```python
from build123d import *

# Parameters (mm, degrees)
SKETCH1_W           = 90
SKETCH1_H           = 70
BOSS_EXTRUDE1_DEPTH = 4
SKETCH2_R           = 1.75
CUT_EXTRUDE1_DEPTH  = 5
CHAMFER1_SIZE       = 2
CHAMFER2_SIZE       = 2
CHAMFER3_SIZE       = 2
CHAMFER4_SIZE       = 2
SKETCH5_W           = 70
SKETCH5_H           = 4
BOSS_EXTRUDE3_DEPTH = 10
SKETCH4_W           = 70
SKETCH4_H           = 4
BOSS_EXTRUDE4_DEPTH = 10
SKETCH6_R           = 1.75
CUT_EXTRUDE2_DEPTH  = 10
CHAMFER5_SIZE       = 2
SKETCH7_W           = 40
SKETCH7_H           = 40
CUT_EXTRUDE3_DEPTH  = 2
SKETCH8_W           = 25
SKETCH8_H           = 15
CUT_EXTRUDE4_DEPTH  = 2
SKETCH9_R           = 1.5
CUT_EXTRUDE5_DEPTH  = 4
SKETCH10_R          = 1.75
CUT_EXTRUDE6_DEPTH  = 10


with BuildPart() as part:
    # Sketch1 → Boss-Extrude1 (new body)
    with BuildSketch(Plane.XY):
        with Locations((44.768273235, 35.193370166)):
            Rectangle(SKETCH1_W, SKETCH1_H)
    extrude(amount=BOSS_EXTRUDE1_DEPTH)

    # Sketch2 → Cut-Extrude1 (cut)
    with BuildSketch(Plane.XY.offset(4)):
        with Locations((3.703568783, 2.693370166)):
            Circle(SKETCH2_R)
        with Locations((86.703568783, 2.694436567)):
            Circle(SKETCH2_R)
        with Locations((86.703273235, 67.693370166)):
            Circle(SKETCH2_R)
        with Locations((3.703273235, 67.693370166)):
            Circle(SKETCH2_R)
        with Locations((23.297725672, 13.693370166)):
            Circle(SKETCH2_R)
        with Locations((66.284051901, 13.693370166)):
            Circle(SKETCH2_R)
        with Locations((66.268273235, 56.693370166)):
            Circle(SKETCH2_R)
        with Locations((23.268273235, 56.693370166)):
            Circle(SKETCH2_R)
    extrude(amount=-CUT_EXTRUDE1_DEPTH, mode=Mode.SUBTRACT)

    # Chamfer1
    chamfer1_edges = [part.edges().sort_by_distance(p)[0] for p in [
        (89.768273235, 0.193370166, 2),
    ]]
    chamfer(chamfer1_edges, length=CHAMFER1_SIZE)

    # Chamfer2
    chamfer2_edges = [part.edges().sort_by_distance(p)[0] for p in [
        (-0.231726765, 0.193370166, 2),
    ]]
    chamfer(chamfer2_edges, length=CHAMFER2_SIZE)

    # Chamfer3
    chamfer3_edges = [part.edges().sort_by_distance(p)[0] for p in [
        (-0.231726765, 70.193370166, 2),
    ]]
    chamfer(chamfer3_edges, length=CHAMFER3_SIZE)

    # Chamfer4
    chamfer4_edges = [part.edges().sort_by_distance(p)[0] for p in [
        (89.768273235, 70.193370166, 2),
    ]]
    chamfer(chamfer4_edges, length=CHAMFER4_SIZE)

    # Sketch5 → Boss-Extrude3 (add)
    with BuildSketch(Plane(origin=(0, 70.193370166, 0), x_dir=(1, 0, 0), z_dir=(0, 1, 0))):
        with Locations((44.768273235, -2)):
            Rectangle(SKETCH5_W, SKETCH5_H)
    extrude(amount=BOSS_EXTRUDE3_DEPTH)

    # Sketch4 → Boss-Extrude4 (add)
    with BuildSketch(Plane(origin=(0, 0.193370166, 0), x_dir=(-1, 0, 0), z_dir=(0, -1, 0))):
        with Locations((-44.768273235, -2)):
            Rectangle(SKETCH4_W, SKETCH4_H)
    extrude(amount=BOSS_EXTRUDE4_DEPTH)

    # Sketch6 → Cut-Extrude2 (cut)
    with BuildSketch(Plane(origin=(0, 0, 0), x_dir=(-1, 0, 0), z_dir=(0, 0, -1))):
        with Locations((-12.268273235, 76.693370166)):
            Circle(SKETCH6_R)
        with Locations((-77.268273235, 76.693370166)):
            Circle(SKETCH6_R)
        with Locations((-77.268273235, -6.306629834)):
            Circle(SKETCH6_R)
        with Locations((-12.268273235, -6.306629834)):
            Circle(SKETCH6_R)
    extrude(amount=-CUT_EXTRUDE2_DEPTH, mode=Mode.SUBTRACT)

    # Chamfer5
    chamfer5_edges = [part.edges().sort_by_distance(p)[0] for p in [
        (9.768273235, 80.193370166, 2),
        (79.768273235, 80.193370166, 2),
        (9.768273235, -9.806629834, 2),
        (79.768273235, -9.806629834, 2),
    ]]
    chamfer(chamfer5_edges, length=CHAMFER5_SIZE)

    # Sketch7 → Cut-Extrude3 (cut)
    with BuildSketch(Plane(origin=(0, 0, 0), x_dir=(-1, 0, 0), z_dir=(0, 0, -1))):
        with Locations((-44.768273235, 35.193370166)):
            Rectangle(SKETCH7_W, SKETCH7_H)
    extrude(amount=-CUT_EXTRUDE3_DEPTH, mode=Mode.SUBTRACT)

    # Sketch8 → Cut-Extrude4 (cut)
    with BuildSketch(Plane(origin=(0, 0, 0), x_dir=(-1, 0, 0), z_dir=(0, 0, -1))):
        with Locations((-77.268273235, 35.193370166)):
            Rectangle(SKETCH8_W, SKETCH8_H)
    extrude(amount=-CUT_EXTRUDE4_DEPTH, mode=Mode.SUBTRACT)

    # Sketch9 → Cut-Extrude5 (cut)
    with BuildSketch(Plane(origin=(0, 0, 0), x_dir=(-1, 0, 0), z_dir=(0, 0, -1))):
        with Locations((-27.768273235, 9.193370166)):
            Circle(SKETCH9_R)
        with Locations((-58.768273235, 9.193370166)):
            Circle(SKETCH9_R)
        with Locations((-27.768273235, 64.193370166)):
            Circle(SKETCH9_R)
        with Locations((-58.768273235, 64.193370166)):
            Circle(SKETCH9_R)
    extrude(amount=-CUT_EXTRUDE5_DEPTH, mode=Mode.SUBTRACT)

    # Sketch10 → Cut-Extrude6 (cut)
    with BuildSketch(Plane(origin=(0, 0, 0), x_dir=(-1, 0, 0), z_dir=(0, 0, -1))):
        with Locations((-74.871589862, 34.731015085)):
            Circle(SKETCH10_R)
        with Locations((-44.465998271, 4.325423494)):
            Circle(SKETCH10_R)
        with Locations((-14.06040668, 34.731015085)):
            Circle(SKETCH10_R)
        with Locations((-44.465998271, 65.136606676)):
            Circle(SKETCH10_R)
    extrude(amount=-CUT_EXTRUDE6_DEPTH, mode=Mode.SUBTRACT)


solid = part.part
```
Work out the finished part from the listing and answer in its coordinate system (mm). A direction names the side the tool comes from. Coordinates: 2 decimals unless noted, no trailing zeros. Loops run counter-clockwise (first coordinate to the right, second up) from the corner with the lowest first, then second, coordinate; pieces in that order, holes last. Notation, with made-up numbers: M -14.75,-31 L 28.25,-31 A18 ccw 28.25,-21 Z; hole C 23.25,20.5 d1. An arc over 180 degrees is marked long. Use CSV: the item, a comma, the result in double quotes. Start each with the question number.
(1) Consider line 1 (X direction, y = 13.5, z = 1); line 2 (X direction, y = 16, z = 1.2); line 3 (X direction, y = 2.5, z = 1.95). Determine where each line is inside the solid, lowest interval first.
(2) Find section A-A, the plane x = 52.5. Give the vertices of the cut face in (y, z).
(3) Find section C-C, the plane x = 71. Give the vertices of the cut face in (y, z).
(4) For faces 1 (the face through (6, 0.193, 2)), 2 (the face through (77, 27.693, 1)), 3 (the face through (45, 55.193, 1)), 4 (the face through (6, 70.193, 2)), determine the directions among +Z, -Z, +X, -X, +Y, -Y from which every point of the face is accessible in a straight line to the end or side of a thin tool.
(5) For a pull along X with two mould halves and no side action, classify faces 5 (the face through (45, 15.193, 1)), 6 (the face through (-0.232, 35, 2)), 7 (the face through (84, 70.193, 2)) as +X half, -X half, draft (parallel to the pull), parting line (faces both ways), or undercut.
(6) Given pin 1 Ø2.5 at (x, y) = (27.77, 9.19) entering from +Z; pin 2 Ø1.2 at (y, z) = (76, 1.5) entering from -X; pin 3 Ø1.2 at (x, z) = (83, 3) entering from -Y; pin 4 Ø12 at (x, y) = (31, 45.5) entering from -Z, each flat-ended and moving along its own axis, determine where each tip first touches the part or whether it passes through.
(7) Find section B-B, the plane y = 41. Give the vertices of the cut face in (x, z), then the cut area to 3 significant figures.
(8) Find section D-D, the plane z = 2.7. State how many separate pieces and enclosed holes the cut face has, then the cut area to 3 significant figures.
Recorded:
1,line 1,"x = -0.23 to 21.56, 25.04 to 64.54, 68.02 to 89.77"
1,line 2,"x = -0.23 to 24.77, 64.77 to 89.77"
1,line 3,"x = -0.23 to 1.96, 5.44 to 84.96, 88.44 to 89.77"
2,outline,"M -9.81,0 L 15.19,0 L 15.19,2 L 55.19,2 L 55.19,0 L 80.19,0 L 80.19,4 L -9.81,4 Z"
3,outline,"M -9.81,0 L 27.69,0 L 27.69,2 L 42.69,2 L 42.69,0 L 80.19,0 L 80.19,4 L -9.81,4 Z"
4,face 1,"+Z, -Z, -X, -Y"
4,face 2,"-Z, +X"
4,face 3,"-Z"
4,face 4,"+Z, -Z, -X, +Y"
5,face 5,"undercut"
5,face 6,"-X half"
5,face 7,"draft"
6,pin 1,"passes through"
6,pin 2,"stops at x = 9.77"
6,pin 3,"stops at y = 0.19"
6,pin 4,"stops at z = 2"
7,outline,"M -0.23,0 L 24.77,0 L 24.77,2 L 89.77,2 L 89.77,4 L -0.23,4 Z"
7,area,"230 mm^2"
8,separate pieces,"1"
8,enclosed holes,"20"
8,area,"7,500 mm^2"
